from build123d import *

# Parameters (mm, degrees)
BOSS_EXTRUDE1_DEPTH = 6.35


with BuildPart() as part:
    # Sketch1 → Boss-Extrude1 (new body)
    with BuildSketch(Plane.XY):
        with BuildLine():
            Line((8823.036740753, 3168.83754785), (8823.036740753, 3119.67584785))
            Line((8823.036740753, 3119.67584785), (8816.051740753, 3119.67584785))
            ThreePointArc((8816.051740753, 3119.67584785), (8813.806676722, 3118.74591188), (8812.876740753, 3116.50084785))
            Line((8812.876740753, 3116.50084785), (8812.876740753, 3106.97584785))
            ThreePointArc((8812.876740753, 3106.97584785), (8813.806676722, 3104.73078382), (8816.051740753, 3103.80084785))
            Line((8816.051740753, 3103.80084785), (8823.036740753, 3103.80084785))
            Line((8823.036740753, 3103.80084785), (8823.036740753, 3095.59664785))
            ThreePointArc((8823.036740753, 3095.59664785), (8820.834652376, 3090.280336226), (8815.518340753, 3088.07824785))
            Line((8815.518340753, 3088.07824785), (8815.518340753, 3091.48184785))
            Line((8815.518340753, 3091.48184785), (8802.818340753, 3091.48184785))
            Line((8802.818340753, 3091.48184785), (8802.818340753, 3088.07824785))
            Line((8802.818340753, 3088.07824785), (8762.229140753, 3088.07824785))
            Line((8762.229140753, 3088.07824785), (8762.229140753, 3091.48184785))
            Line((8762.229140753, 3091.48184785), (8749.529140753, 3091.48184785))
            Line((8749.529140753, 3091.48184785), (8749.529140753, 3088.07824785))
            ThreePointArc((8749.529140753, 3088.07824785), (8744.212829129, 3090.280336226), (8742.010740753, 3095.59664785))
            Line((8742.010740753, 3095.59664785), (8742.010740753, 3103.80084785))
            Line((8742.010740753, 3103.80084785), (8748.995740753, 3103.80084785))
            ThreePointArc((8748.995740753, 3103.80084785), (8751.240804783, 3104.73078382), (8752.170740753, 3106.97584785))
            Line((8752.170740753, 3106.97584785), (8752.170740753, 3116.50084785))
            ThreePointArc((8752.170740753, 3116.50084785), (8751.240804783, 3118.74591188), (8748.995740753, 3119.67584785))
            Line((8748.995740753, 3119.67584785), (8742.010740753, 3119.67584785))
            Line((8742.010740753, 3119.67584785), (8742.010740753, 3168.83754785))
            Line((8742.010740753, 3168.83754785), (8747.090740753, 3168.83754785))
            Line((8747.090740753, 3168.83754785), (8747.090740753, 3194.23754785))
            Line((8747.090740753, 3194.23754785), (8749.529140753, 3194.23754785))
            Line((8749.529140753, 3194.23754785), (8749.529140753, 3190.83394785))
            Line((8749.529140753, 3190.83394785), (8762.229140753, 3190.83394785))
            Line((8762.229140753, 3190.83394785), (8762.229140753, 3194.23754785))
            Line((8762.229140753, 3194.23754785), (8802.818340753, 3194.23754785))
            Line((8802.818340753, 3194.23754785), (8802.818340753, 3190.83394785))
            Line((8802.818340753, 3190.83394785), (8815.518340753, 3190.83394785))
            Line((8815.518340753, 3190.83394785), (8815.518340753, 3194.23754785))
            Line((8815.518340753, 3194.23754785), (8817.956740753, 3194.23754785))
            Line((8817.956740753, 3194.23754785), (8817.956740753, 3168.83754785))
            Line((8817.956740753, 3168.83754785), (8823.036740753, 3168.83754785))
        make_face()
        with BuildLine():
            Line((8780.603057309, 3143.88204785), (8753.948740753, 3143.88204785))
            Line((8753.948740753, 3143.88204785), (8753.948740753, 3148.04764785))
            Line((8753.948740753, 3148.04764785), (8811.098740753, 3148.04764785))
            Line((8811.098740753, 3148.04764785), (8811.098740753, 3143.88204785))
            Line((8811.098740753, 3143.88204785), (8784.444424196, 3143.88204785))
            ThreePointArc((8784.444424196, 3143.88204785), (8784.419103776, 3143.858656943), (8784.440418599, 3143.831565681))
            ThreePointArc((8784.440418599, 3143.831565681), (8782.523740753, 3119.67584785), (8780.607062906, 3143.831565681))
            ThreePointArc((8780.607062906, 3143.831565681), (8780.628377729, 3143.858656943), (8780.603057309, 3143.88204785))
        make_face(mode=Mode.SUBTRACT)
    extrude(amount=BOSS_EXTRUDE1_DEPTH)


solid = part.part
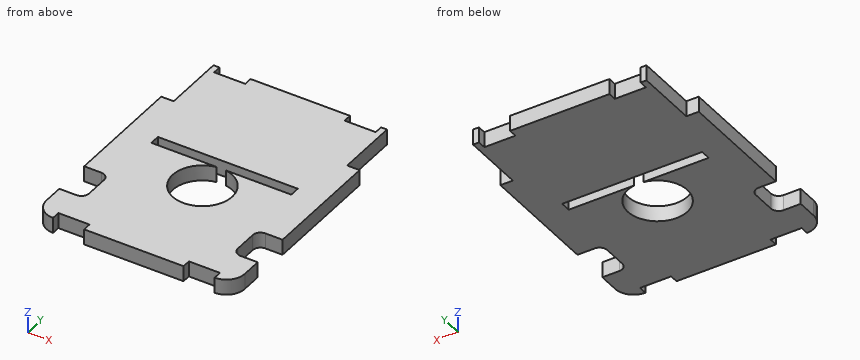
The listing builds one solid part. Answer for the finished solid, in the listing's coordinates (mm). Round coordinates to 2 decimals unless told otherwise and drop trailing zeros. Order: outer loops, then holes, each group sorted by start corner. A loop starts at its lowest first (then second) coordinate and runs counter-clockwise, first axis right, second up. Notation, with made-up numbers: (-18.5, 45.5) - (19.5, 45.5) arc R26 ccw to (19.5, 61.5) - close; hole circle Ø2 at (30, 69.5). An arc over 180 degrees is marked (long way). Write item = value, one per line. Start each with the question number.
1) Section A-A, the plane x = 8760.5 is taken. Write down the section's boundary in (y, z).
2) Section B-B, the plane y = 3141 is taken. Write down the section's boundary in (x, z), plus the area to 3 significant figures.
3) Section C-C, the plane x = 8787 is taken. Write down the section's boundary in (y, z).
4) Given pin 1 (3.5 mm diameter, centred on y = 3089, z = 3, fed in from -X); pin 2 (1 mm diameter, centred on y = 3090, z = 2.5, fed in from +X); pin 3 (1 mm diameter, centred on y = 3090.5, z = 3.5, fed in from -X), each flat-ended and moving along its own axis, determine where each tip first touches the part or whether it passes through.
5) Section D-D, the plane y = 3171 is taken. Write down the section's boundary in (x, z), plus the area to 3 significant figures.
6) Straight lines are drawn through the part: L1, parallel to Y at x = 8766, z = 1.75; L2, parallel to Y at x = 8772, z = 5.25; L3, parallel to Y at x = 8758.5, z = 3.5. For each, find the intervals that lie inside material, in ascending order.
Results list:
q1.outline = (3091.48, 0) - (3143.88, 0) - (3143.88, 6.35) - (3091.48, 6.35) - close; (3148.05, 0) - (3190.83, 0) - (3190.83, 6.35) - (3148.05, 6.35) - close
q2.outline = (8742.01, 0) - (8774.55, 0) - (8774.55, 6.35) - (8742.01, 6.35) - close; (8790.5, 0) - (8823.04, 0) - (8823.04, 6.35) - (8790.5, 6.35) - close
q2.area = 413 mm^2
q3.outline = (3088.08, 0) - (3120.53, 0) - (3120.53, 6.35) - (3088.08, 6.35) - close; (3143.13, 0) - (3143.88, 0) - (3143.88, 6.35) - (3143.13, 6.35) - close; (3148.05, 0) - (3194.24, 0) - (3194.24, 6.35) - (3148.05, 6.35) - close
q4.pin_1 = 8743.78
q4.pin_2 = 8821.05
q4.pin_3 = 8743.58
q5.outline = (8747.09, 0) - (8817.96, 0) - (8817.96, 6.35) - (8747.09, 6.35) - close
q5.area = 450 mm^2
q6.L1 = 3088.08 to 3143.88, 3148.05 to 3194.24
q6.L2 = 3088.08 to 3125.75, 3137.91 to 3143.88, 3148.05 to 3194.24
q6.L3 = 3091.48 to 3143.88, 3148.05 to 3190.83
